```python
from build123d import *
from build123d import SkipClean  # not in build123d's __all__

# Parameters (mm, degrees)
F0_R     = 8.5
F1_DEPTH = 15
F2_R     = 1.5
F4_R     = 2
F5_DEPTH = 5
F7_DEPTH = 5


with BuildPart() as f1:
    # F0 (on Top) → F1 (new body)
    with BuildSketch(Plane.XY):
        with BuildLine():
            Line((-32.5, -22), (-32.5, 22))
            ThreePointArc((-32.5, 22), (-41.2620999228, 0), (-32.5, -22))
        make_face()
        with BuildLine():
            ThreePointArc((32.5, 22), (0, 14.592529173), (-32.5, 22))
            Line((-32.5, 22), (0, 0))
            Line((0, 0), (32.5, 22))
        make_face()
        Polygon((0, 0), (-32.5, 22), (-32.5, -22), align=None)
        with BuildLine():
            Line((0, 0), (-32.5, -22))
            ThreePointArc((-32.5, -22), (-19.5807119119, -17.1936637052), (-6, -14.8329144067))
            ThreePointArc((-6, -14.8329144067), (0, -14.592529173), (6, -14.8329144067))
            ThreePointArc((6, -14.8329144067), (19.5807119119, -17.1936637052), (32.5, -22))
            Line((32.5, -22), (0, 0))
        make_face()
        Polygon((32.5, -22), (32.5, 22), (0, 0), align=None)
        with BuildLine():
            ThreePointArc((32.5, -22), (41.2620999228, 0), (32.5, 22))
            Line((32.5, 22), (32.5, -22))
        make_face()
        with BuildLine():
            ThreePointArc((6, -14.8329144067), (0, -14.592529173), (-6, -14.8329144067))
            Line((-6, -14.8329144067), (-6, -74.8329144067))
            Line((-6, -74.8329144067), (6, -74.8329144067))
            Line((6, -74.8329144067), (6, -14.8329144067))
        make_face()
        with BuildLine():
            Line((6, -74.8329144067), (-6, -74.8329144067))
            ThreePointArc((-6, -74.8329144067), (0, -102.5332931892), (6, -74.8329144067))
        make_face()
        with Locations((0, -88.0332931892)):
            Circle(F0_R, mode=Mode.SUBTRACT)
    extrude(amount=F1_DEPTH)

    # F2
    f2_edges = [f1.edges().sort_by_distance(p)[0] for p in [
        (-6, -44.832914, 15),
        (6, -44.832914, 15),
        (6, -44.832914, 0),
        (-6, -44.832914, 0),
    ]]
    fillet(f2_edges, radius=F2_R)

    # F4
    f4_edges = [f1.edges().sort_by_distance(p)[0] for p in [
        (-19.580712, -17.193664, 15),
        (-41.2621, 0, 15),
        (19.580712, -17.193664, 15),
        (-19.580712, -17.193664, 0),
        (-41.2621, 0, 0),
        (0, 14.592529, 0),
        (41.2621, 0, 0),
        (19.580712, -17.193664, 0),
        (41.2621, 0, 15),
        (0, 14.592529, 15),
    ]]
    fillet(f4_edges, radius=F4_R)

    # F3 (on face) → F5 (cut)
    with BuildSketch(Plane.XY.offset(15)):
        with BuildLine():
            Line((-29.3147544782, -16.5), (-29.3147544782, 16.5))
            ThreePointArc((-29.3147544782, 16.5), (-38.0120999228, 0), (-29.3147544782, -16.5))
        make_face()
        with BuildLine():
            ThreePointArc((0, 11.342529173), (-14.8824925286, 12.6417227993), (-29.3147544782, 16.5))
            Line((-29.3147544782, 16.5), (0, 0))
            Line((0, 0), (0, 11.342529173))
        make_face()
        Polygon((0, 0), (-29.3147544782, 16.5), (-29.3147544782, -16.5), align=None)
        with BuildLine():
            Line((0, 0), (-29.3147544782, -16.5))
            ThreePointArc((-29.3147544782, -16.5), (-14.8824925285, -12.6417227993), (0, -11.342529173))
            Line((0, -11.342529173), (0, 0))
        make_face()
        with BuildLine():
            ThreePointArc((29.3147544782, 16.5), (14.8824925286, 12.6417227993), (0, 11.342529173))
            Line((0, 11.342529173), (0, 0))
            Line((0, 0), (29.3147544782, 16.5))
        make_face()
        Polygon((29.3147544782, 16.5), (0, 0), (29.3147544782, -16.5), align=None)
        with BuildLine():
            Line((29.3147544782, -16.5), (0, 0))
            Line((0, 0), (0, -11.342529173))
            ThreePointArc((0, -11.342529173), (14.8824925286, -12.6417227993), (29.3147544782, -16.5))
        make_face()
        with BuildLine():
            ThreePointArc((29.3147544782, -16.5), (38.0120999228, 0), (29.3147544782, 16.5))
            Line((29.3147544782, 16.5), (29.3147544782, -16.5))
        make_face()
    with SkipClean():  # cleaning this boolean's faces spoils the solid; the shape is the same uncleaned
        extrude(amount=-F5_DEPTH, mode=Mode.SUBTRACT)

    # F6 (on face) → F7 (join)
    with BuildSketch(Plane.XY.offset(10)):
        with BuildLine():
            Line((15.2079802839, 12.699633284), (11.3304843403, -12.0931563405))
            ThreePointArc((11.3304843403, -12.0931563405), (13.3952654965, -12.3935064492), (15.4521416161, -12.7439233999))
            Line((15.4521416161, -12.7439233999), (17.8190562874, 0))
            Line((17.8190562874, 0), (22.0686495304, -1.6748139169))
            Line((22.0686495304, -1.6748139169), (24.2379181726, -14.8333900519))
            ThreePointArc((24.2379181726, -14.8333900519), (26.7892998078, -15.6272055953), (29.3147544782, -16.5))
            Line((29.3147544782, -16.5), (22.4350078947, 14.3243580948))
            ThreePointArc((22.4350078947, 14.3243580948), (18.8390172894, 13.4340497811), (15.2079802839, 12.699633284))
        make_face()
        Polygon((17.8190562874, 4.6145855449), (19.5188932121, 10.9039852396), (21.3887151331, 2.9147479217), align=None, mode=Mode.SUBTRACT)
        with BuildLine():
            Line((-2.0585943572, 11.3672025947), (-6.3891717286, -11.5804961029))
            ThreePointArc((-6.3891717286, -11.5804961029), (1.0259296068, -11.3486565705), (8.4333769686, -11.7575587165))
            Line((8.4333769686, -11.7575587165), (7.4048662885, -7.905074934))
            Line((7.4048662885, -7.905074934), (0, -6.9299801253))
            Line((0, -6.9299801253), (2.4106339203, 11.3763647448))
            ThreePointArc((2.4106339203, 11.3763647448), (0.1760793848, 11.3427096587), (-2.0585943572, 11.3672025947))
        make_face()
        with BuildLine():
            ThreePointArc((-29.3147544782, 16.5), (-30.604070915, 15.5384126129), (-31.8119491831, 14.4763310404))
            Line((-31.8119491831, 14.4763310404), (-24.5027556892, -14.9117551872))
            ThreePointArc((-24.5027556892, -14.9117551872), (-22.5955271512, -14.3679613691), (-20.6762515008, -13.8683481283))
            Line((-20.6762515008, -13.8683481283), (-19.114445895, -6.066611968))
            Line((-19.114445895, -6.066611968), (-17.2392854565, -13.0903846112))
            ThreePointArc((-17.2392854565, -13.0903846112), (-14.7242186042, -12.614029589), (-12.1960735351, -12.2128340149))
            Line((-12.1960735351, -12.2128340149), (-9.0315309989, 11.8186900319))
            ThreePointArc((-9.0315309989, 11.8186900319), (-10.8625432372, 12.0321900371), (-12.6885517924, 12.2849366013))
            Line((-12.6885517924, 12.2849366013), (-16.3512527943, -6.066611968))
            Line((-16.3512527943, -6.066611968), (-17.7929196507, 7.7493544668))
            Line((-17.7929196507, 7.7493544668), (-20.6762515008, 4.6145855449))
            Line((-20.6762515008, 4.6145855449), (-21.8776389956, -6.066611968))
            Line((-21.8776389956, -6.066611968), (-27.7557073698, 15.9508191787))
            ThreePointArc((-27.7557073698, 15.9508191787), (-28.5365520654, 16.2216590548), (-29.3147544782, 16.5))
        make_face()
    with SkipClean():  # cleaning this boolean's faces spoils the solid; the shape is the same uncleaned
        extrude(amount=F7_DEPTH)


solid = f1.part
```
Source: CAD feature listing. Evaluate the final solid. Frame: model axes, mm. A direction names the side the tool comes from. Round coordinates to 2 decimals unless told otherwise and drop trailing zeros. Loops run counter-clockwise (first coordinate to the right, second up) from the corner with the lowest first, then second, coordinate; pieces in that order, holes last. Notation, with made-up numbers: (22, 61) - (56, 61) arc R23 ccw to (56, 97) - close; hole circle Ø3 at (-37.75, -22). An arc over 180 degrees is marked (long way). Use CSV: the item, a comma, the result in double quotes.
Q1. Reachability of faces 1 (the flat face through (-7, 0, 10)), 2 (the flat face through (-1, -13, 0)) from +Z, -Z, +X, -X, +Y, -Y: full face, straight path, thin tool, end or side. Return the list, or none.
Reported:
face 1,"+Z"
face 2,"-Z, +X, -X, +Y, -Y"
Q2. Section query B-B, the plane z = 6. Output: boundary loops of the cut face in (x, y), then the cut area to 3 significant figures.
Reported:
outline,"(-32.5, -22) arc R75 cw to (-6, -14.83) - (-6, -74.83) arc R14.5 ccw (long way) to (6, -74.83) - (6, -14.83) arc R75 cw to (32.5, -22) arc R32 ccw to (32.5, 22) arc R75 cw to (-32.5, 22) arc R32 ccw to start; hole circle Ø17 at (0, -88.03)"
area,"3,890 mm^2"
Q3. Section query A-A, the plane y = -90.5. Output: boundary loops of the cut face in (x, z), then the cut area to 3 significant figures.
Reported:
outline,"(-14.29, 0) - (-8.13, 0) - (-8.13, 15) - (-14.29, 15) - close; (8.13, 0) - (14.29, 0) - (14.29, 15) - (8.13, 15) - close"
area,"185 mm^2"
Q4. Section query C-C, the plane y = -51. Output: boundary loops of the cut face in (x, z), then the cut area to 3 significant figures.
Reported:
outline,"(-6, 1.5) arc R1.5 ccw to (-4.5, 0) - (4.5, 0) arc R1.5 ccw to (6, 1.5) - (6, 13.5) arc R1.5 ccw to (4.5, 15) - (-4.5, 15) arc R1.5 ccw to (-6, 13.5) - close"
area,"178 mm^2"
Q5. Pin query (flat end, axial travel): pin 1 Ø8 at (x, y) = (-6, -5) entering from +Z; pin 2 Ø4.5 at (x, y) = (5.5, 4.5) entering from +Z; pin 3 Ø2 at (x, z) = (-26.5, 13) entering from -Y; pin 4 Ø1.5 at (y, z) = (-26, 4) entering from -X. Return the tip coordinate at first contact, or that it passes through.
Reported:
pin 1,"z = 15"
pin 2,"z = 10"
pin 3,"y = -19.82"
pin 4,"x = -6"
Q6. Ray query, line 1 along Y through (x, z) = (0, 5.25); line 2 along Y through (x, z) = (-7, 1); line 3 along Y through (x, z) = (-36, 13.5). Return the intervals inside material, ascending.
Reported:
line 1,"-102.53 to -96.53, -79.53 to 14.59"
line 2,"-100.73 to -92.86, -83.21 to -75.33, -14.65 to 14.65"
line 3,"-17.46 to -8.74, 8.74 to 17.46"
Q7. Mould query, pull axis Y, two halves, no side actions, for faces 3 (the flat face through (3.754, -7.424, 12.465)), 4 (the flat face through (0, -32, 15)), 5 (the flat face through (23.138, -8.162, 12.465)). Classes: pulls with the +Y half, pulls with the -Y half, needs draft (parallel to the pull), parting line crosses it, or undercut.
Reported:
face 3,"undercut"
face 4,"needs draft"
face 5,"undercut"
